```python
from build123d import *

# Parameters (mm, degrees)
SKETCH1_R           = 11.162804955
BOSS_EXTRUDE1_DEPTH = 25.4
BOSS_EXTRUDE2_START = -2.54
BOSS_EXTRUDE2_DEPTH = 2.54
SKETCH4_W           = 66.04
SKETCH4_H           = 25.4
BOSS_EXTRUDE3_DEPTH = 16.064370514
SKETCH5_W           = 1.129641984
SKETCH5_H           = 25.4
BOSS_EXTRUDE4_DEPTH = 38.1
SKETCH6_W           = 26.67
SKETCH6_H           = 25.4
BOSS_EXTRUDE5_DEPTH = 16.461081374
BOSS_EXTRUDE8_DEPTH = 2.54


with BuildPart() as part:
    # Sketch1 → Boss-Extrude1 (new body)
    with BuildSketch(Plane.XY):
        Circle(SKETCH1_R)
    extrude(amount=-BOSS_EXTRUDE1_DEPTH)

    # Sketch2 → Boss-Extrude2 (add)
    with BuildSketch(Plane(origin=(0, 0, -25.4), x_dir=(-1, 0, 0), z_dir=(0, 0, -1)).offset(BOSS_EXTRUDE2_START)):
        with BuildLine():
            Line((-11.162804955, 0), (-11.162804955, 25.4))
            Line((-11.162804955, 25.4), (11.162804955, 25.4))
            Line((11.162804955, 25.4), (11.162804955, 0))
            ThreePointArc((11.162804955, 0), (0, 11.162804955), (-11.162804955, 0))
        make_face()
    extrude(amount=BOSS_EXTRUDE2_DEPTH)

    # Sketch4 → Boss-Extrude3 (add)
    with BuildSketch(Plane(origin=(0, 25.4, 0), x_dir=(1, 0, 0), z_dir=(0, 1, 0))):
        with Locations((0, 12.7)):
            Rectangle(SKETCH4_W, SKETCH4_H)
    extrude(amount=BOSS_EXTRUDE3_DEPTH)

    # Sketch5 → Boss-Extrude4 (add)
    with BuildSketch(Plane(origin=(0, 41.464370514, 0), x_dir=(1, 0, 0), z_dir=(0, 1, 0))):
        with Locations((-32.455179008, 12.7)):
            Rectangle(SKETCH5_W, SKETCH5_H)
        with Locations((32.455179008, 12.7)):
            Rectangle(SKETCH5_W, SKETCH5_H)
    extrude(amount=BOSS_EXTRUDE4_DEPTH)

    # Sketch6 → Boss-Extrude5 (add)
    with BuildSketch(Plane(origin=(0, 79.564370514, 0), x_dir=(1, 0, 0), z_dir=(0, 1, 0))):
        with Locations((19.685, 12.7)):
            Rectangle(SKETCH6_W, SKETCH6_H)
        with Locations((-19.685, 12.7)):
            Rectangle(SKETCH6_W, SKETCH6_H)
    extrude(amount=BOSS_EXTRUDE5_DEPTH)

    # Sketch10 → Boss-Extrude8 (add)
    with BuildSketch(Plane(origin=(0, 0, -25.4), x_dir=(-1, 0, 0), z_dir=(0, 0, -1))):
        with BuildLine():
            Line((11.162804955, 0), (11.162804955, 25.4))
            Line((11.162804955, 25.4), (33.02, 25.4))
            Line((33.02, 25.4), (33.02, 96.025451888))
            Line((33.02, 96.025451888), (6.35, 96.025451888))
            Line((6.35, 96.025451888), (6.35, 79.564370514))
            Line((6.35, 79.564370514), (31.890358016, 79.564370514))
            Line((31.890358016, 79.564370514), (31.890358016, 41.464370514))
            Line((31.890358016, 41.464370514), (-31.890358016, 41.464370514))
            Line((-31.890358016, 41.464370514), (-31.890358016, 79.564370514))
            Line((-31.890358016, 79.564370514), (-6.35, 79.564370514))
            Line((-6.35, 79.564370514), (-6.35, 96.025451888))
            Line((-6.35, 96.025451888), (-33.02, 96.025451888))
            Line((-33.02, 96.025451888), (-33.02, 25.4))
            Line((-33.02, 25.4), (-11.162804955, 25.4))
            Line((-11.162804955, 25.4), (-11.162804955, 0))
            ThreePointArc((-11.162804955, 0), (0, -11.162804955), (11.162804955, 0))
        make_face()
    extrude(amount=BOSS_EXTRUDE8_DEPTH)


solid = part.part
```
For this review, take the finished solid that the model builds, in its own axes (mm). A direction names the side the tool comes from. Round coordinates to 2 decimals unless told otherwise and drop trailing zeros. Write each loop counter-clockwise with the first axis right and the second up, starting at its lowest first coordinate (ties: lowest second). Pieces come first, ordered by that corner, then holes. Notation, with made-up numbers: (12, 48) - (49, 48) arc R3 cw to (49, 52) - close; hole circle Ø2 at (34, -38). An arc over 180 degrees is marked (long way). Answer as a JSON object with one key per item and string values.
1. We need section C-C on z = -7.75. Give the boundary of the cut face in (x, y), then the cut area to 3 significant figures.
Response values:
{"outline": "(-33.02, 25.4) - (33.02, 25.4) - (33.02, 96.03) - (6.35, 96.03) - (6.35, 79.56) - (31.89, 79.56) - (31.89, 41.46) - (-31.89, 41.46) - (-31.89, 79.56) - (-6.35, 79.56) - (-6.35, 96.03) - (-33.02, 96.03) - close; circle Ø22.33 at (0, 0)", "area": "2,420 mm2"}
2. For pin 1 Ø1.3 at (y, z) = (16.5, -24) entering from +X; pin 2 Ø3 at (x, y) = (1.5, 16) entering from +Z; pin 3 Ø3 at (x, z) = (15, -23.5) entering from -Y, all flat-tipped, find the tip position at first contact; note any pin that passes through.
Response values:
{"pin 1": "stops at x = 11.16", "pin 2": "stops at z = -22.86", "pin 3": "stops at y = 25.4"}
3. We need section A-A on y = 84. Give the boundary of the cut face in (x, z).
Response values:
{"outline": "(-33.02, -27.94) - (-6.35, -27.94) - (-6.35, 0) - (-33.02, 0) - close; (6.35, -27.94) - (33.02, -27.94) - (33.02, 0) - (6.35, 0) - close"}
4. We need section B-B on x = -18. Give the boundary of the cut face in (y, z).
Response values:
{"outline": "(25.4, -27.94) - (41.46, -27.94) - (41.46, 0) - (25.4, 0) - close; (79.56, -27.94) - (96.03, -27.94) - (96.03, 0) - (79.56, 0) - close"}
5. Draft analysis for pull direction Y (two halves, no side actions). For faces 1 (the face through (0, 19, -22.86)), 2 (the face through (0, 39, -27.94)), state which applies: +Y half, -Y half, draft (parallel to the pull), parting line (faces both ways), or undercut.
Response values:
{"face 1": "undercut", "face 2": "draft"}
6. We need section D-D on x = 0. Give the boundary of the cut face in (y, z).
Response values:
{"outline": "(-11.16, -27.94) - (41.46, -27.94) - (41.46, 0) - (25.4, 0) - (25.4, -22.86) - (11.16, -22.86) - (11.16, 0) - (-11.16, 0) - close"}
7. To check wall thickness, follow line 1 along Y through (x, z) = (-29, -8.5); line 2 along X through (y, z) = (53, -3.25); line 3 along X through (y, z) = (89.5, -21.75). State the ranges of each line that lie inside material, in increasing order.
Response values:
{"line 1": "y = 25.4 to 41.46, 79.56 to 96.03", "line 2": "x = -33.02 to -31.89, 31.89 to 33.02", "line 3": "x = -33.02 to -6.35, 6.35 to 33.02"}
8. Tool access review of faces 3 (the face through (0, 0, 0)), 4 (the face through (-11.163, 13, -25)): name each direction out of +Z, -Z, +X, -X, +Y, -Y from which nothing blocks a thin tool from reaching the whole face with its end or side.
Response values:
{"face 3": "+Z, +X, -X, +Y, -Y", "face 4": "+Z, -Z, -X, -Y"}
